Model file for the job. Use its own axes, mm. Face numbers are marked on the shaded views. A direction names the side the tool comes from. Give positions to 0.01 mm unless a question says otherwise; leave off trailing zeros. Use CSV: the item, a comma, the result in double quotes. Start each with the question number.
(1) Drop flat-ended pins along their axis: pin 1 Ø3 at (x, z) = (-15.5, 0) entering from -Y; pin 2 Ø3 at (x, z) = (-95, 0) entering from +Y; pin 3 Ø5 at (y, z) = (5, 55) entering from -X; pin 4 Ø1 at (x, y) = (-49.5, 4) entering from -Z. Give the stop position or say it passes through.
(2) Tool access for the marked faces 3 and 4: list every direction of +Z, -Z, +X, -X, +Y, -Y with a clear straight run to the whole face (end or side of a thin tool).
(3) Band-saw the part on A-A, the plane y = 9.5. Count the separate pieces of the cut face and the enclosed holes in it, then the cut area to 3 significant figures.
(4) Probe L1, parallel to Z at x = 0, y = 4.5; L2, parallel to X at y = 6, z = 3; L3, parallel to X at y = 5.75, z = -67. List the from-to ranges inside material, lowest first.
(5) Pull direction Z, two halves, no side cores. Call the marked faces 1 and 2: +Z half, -Z half, draft (parallel to the pull), parting line (faces both ways), or undercut.
from build123d import *

# Parameters (mm, degrees)
KES_EKSTR_ZYON3_DEPTH      = 142.972708645
KES_EKSTR_ZYON3_DEPTH_BACK = 142.972708645
IZIM3_R                    = 3.5
IZIM3_R_2                  = 1.75
IZIM4_R                    = 1.4
KES_EKSTR_ZYON4_DEPTH      = 142.972708645
DAIRESEL_KAPLAMA1_COUNT    = 6


with BuildPart() as part:
    # Çizim2 → Döndür1 (revolve)
    with BuildSketch(Plane(origin=(0, 0, 0), x_dir=(0, 0, -1), z_dir=(1, 0, 0))):
        Polygon((0, 0), (-100, 0), (-100, 12.25), (-90.5, 12.25), (-90.5, 2), (-80, 2), (-80, 12.25), (-65, 12.25), (-58, 5), (-37, 5), (-30, 12.5), (0, 12.5), align=None)
    revolve(axis=Axis((0, 27.631034793, 0), (0, -1, 0)))

    # Çizim3 → Kes-Ekstrüzyon3 (cut, two sides: drawn at the far end of the back side and taken through both)
    with BuildSketch(Plane(origin=(0, 12.5, 0), x_dir=(1, 0, 0), z_dir=(0, 1, 0)).offset(-KES_EKSTR_ZYON3_DEPTH_BACK)):
        with Locations(Location((0, 0, 0), (0, 0, 270))):
            Circle(IZIM3_R)
        with Locations(Location((-15.5, 0, 0), (0, 0, 270))):
            Circle(IZIM3_R_2)
        with Locations(Location((0, -15.5, 0), (0, 0, 270))):
            Circle(IZIM3_R_2)
        with Locations(Location((0, 15.5, 0), (0, 0, 270))):
            Circle(IZIM3_R_2)
        with Locations(Location((15.5, 0, 0), (0, 0, 270))):
            Circle(IZIM3_R_2)
    extrude(amount=KES_EKSTR_ZYON3_DEPTH + KES_EKSTR_ZYON3_DEPTH_BACK, mode=Mode.SUBTRACT)

    # Çizim4 → Kes-Ekstrüzyon4 (cut, symmetric)
    with BuildSketch(Plane(origin=(0, 12.5, 0), x_dir=(1, 0, 0), z_dir=(0, 1, 0))):
        with Locations(Location((-75, 0, 0), (0, 0, 270))):
            Circle(IZIM4_R)
        with Locations(Location((-95, 0, 0), (0, 0, 270))):
            Circle(IZIM4_R)
    kes_ekstr_zyon4 = extrude(amount=KES_EKSTR_ZYON4_DEPTH, both=True, mode=Mode.SUBTRACT)

    # Dairesel Kaplama1: Kes-Ekstrüzyon4 ×6 about axis
    dairesel_kaplama1_axis = Axis((0, 0, 0), (0, 1, 0))
    for i in range(1, DAIRESEL_KAPLAMA1_COUNT):
        add(kes_ekstr_zyon4.rotate(dairesel_kaplama1_axis, i * 360 / DAIRESEL_KAPLAMA1_COUNT), mode=Mode.SUBTRACT)


solid = part.part
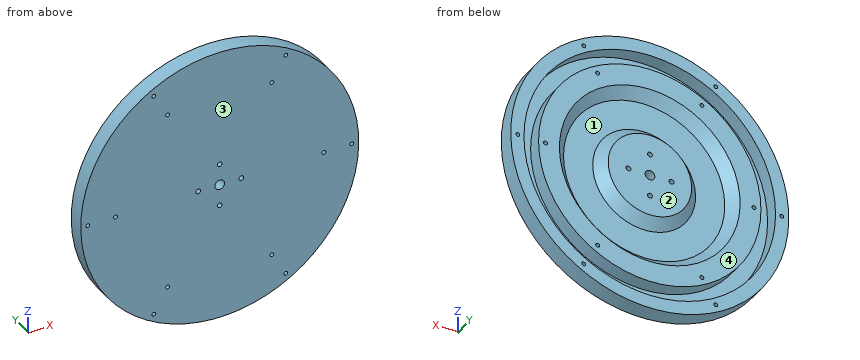
Answer block:
1,pin 1,"passes through"
1,pin 2,"stops at y = 12.25"
1,pin 3,"stops at x = -85.11"
1,pin 4,"stops at z = -87.17"
2,face 3,"+Z, -Z, +X, -X, -Y"
2,face 4,"+Y"
3,separate pieces,"3"
3,enclosed holes,"19"
3,area,"16,800 mm2"
4,L1,"z = -100 to -90.5, -80 to -17.25, -13.75 to -3.5, 3.5 to 13.75, 17.25 to 80, 90.5 to 100"
4,L2,"x = -99.95 to -90.45, -79.94 to -58.89, -35.94 to -1.8, 1.8 to 35.94, 58.89 to 79.94, 90.45 to 99.95"
4,L3,"x = -74.24 to -60.84, -43.71 to 43.71, 60.84 to 74.24"
5,face 1,"undercut"
5,face 2,"draft"
